Work out the finished part from the listing and answer in its coordinate system (mm). A direction names the side the tool comes from. Coordinates: 2 decimals unless noted, no trailing zeros. Write each loop counter-clockwise with the first axis right and the second up, starting at its lowest first coordinate (ties: lowest second). Pieces come first, ordered by that corner, then holes. Notation, with made-up numbers: (8, -37) - (30, -37) arc R13 cw to (30, -13) - close; hole circle Ø7 at (45, -7.75). An arc over 180 degrees is marked (long way). Use one line per item in the form item = value. Start each with the question number.
Item 1: A cutting plane is placed at B-B (z = 30). Write down the section's boundary in (x, y).
Item 2: Determine the mould class of faces 1 (the cylindrical face through (25.879, 48.412, 56.766)), 2 (the flat face through (36, 30.667, 5)), 3 (the cylindrical face through (26.91, 48.41, 2.12)) for opening direction X: released by +X, released by -X, zero draft, split by the parting line, or undercut.
Item 3: Given pin 1 (1.4 mm diameter, centred on y = 45, z = 51, fed in from +X); pin 2 (12 mm diameter, centred on y = 49, z = 39, fed in from +X); pin 3 (8 mm diameter, centred on x = 50, y = 36.5, fed in from -Z), each flat-ended and moving along its own axis, determine where each tip first touches the part or whether it passes through.
Item 4: For faces 4 (the flat face through (16.534, 48, 51)), 5 (the flat face through (36, 65.667, 5)), determine the directions among +Z, -Z, +X, -X, +Y, -Y from which every point of the face is accessible in a straight line to the end or side of a thin tool.
Item 5: Consider probe 1 along Z at (x, y) = (29.5, 34.5); probe 2 along Z at (x, y) = (23.5, 40); probe 3 along X at (y, z) = (38, 32). Determine where each line is inside the solid, lowest interval first.
Item 6: A cutting plane is placed at A-A (x = 40). Write down the section's boundary in (y, z).
from build123d import *

# Parameters (mm, degrees)
SKETCH_1_R      = 25.5
EXTRUDE_1_DEPTH = 35
CHAMFER_1_SIZE  = 1.5
FILLET_1_R      = 2
CHAMFER_2_SIZE  = 0.5


with BuildPart() as part:
    # Эскиз1 → Бобышка-Вытянуть1 (new body)
    # profile 1 of 3: a face of its own
    with BuildSketch(Plane(origin=(0, 65.667309681, 0), x_dir=(-1, 0, 0), z_dir=(0, -1, 0))):
        with BuildLine():
            ThreePointArc((-32.569554052, -57.83154498), (-26.905120992, -2.121558707), (-31.457793139, -57.933399285))
            Line((-31.457793139, -57.933399285), (-31.386430924, -56.935948818))
            ThreePointArc((-31.386430924, -56.935948818), (-26.058947255, -56.789767316), (-20.863962526, -55.599983748))
            Line((-20.863962526, -55.599983748), (-21.100431285, -54.895855797))
            ThreePointArc((-21.100431285, -54.895855797), (-26.672454195, -56.113662764), (-32.375987665, -56.099553559))
            Line((-32.375987665, -56.099553559), (-32.569554052, -57.83154498))
        make_face()
        with Locations((-29.45965114, -30.004786206)):
            Circle(SKETCH_1_R, mode=Mode.SUBTRACT)
    # profile 2 of 3: a face of its own
    with BuildSketch(Plane(origin=(0, 65.667309681, 0), x_dir=(-1, 0, 0), z_dir=(0, -1, 0))):
        with BuildLine():
            ThreePointArc((-42.146247167, -7.884653267), (-43.001975074, -8.397947879), (-43.836965332, -8.944329501))
            Line((-43.836965332, -8.944329501), (-42.312872357, -9.648278017))
            Line((-42.312872357, -9.648278017), (-42.146247167, -7.884653267))
        make_face()
    # profile 3 of 3: a face of its own
    with BuildSketch(Plane(origin=(0, 65.667309681, 0), x_dir=(-1, 0, 0), z_dir=(0, -1, 0))):
        with BuildLine():
            Line((-16.534234919, -50.219751552), (-16.534234919, -51.986224182))
            ThreePointArc((-16.534234919, -51.986224182), (-15.879111186, -51.587625096), (-15.236269322, -51.169507079))
            Line((-15.236269322, -51.169507079), (-16.534234919, -50.219751552))
        make_face()
    extrude(amount=EXTRUDE_1_DEPTH)

    # Фаска1
    # the kernel refuses this chamfer: 1.5 mm, written as the material it takes off along each edge
    with BuildSketch(Plane(origin=(32.569554052, 69.524834163, 57.83154498), x_dir=(0.9905736381961588, 0, -0.13698126627690838), z_dir=(0, -1, 0))) as chamfer_1_piece_1:
        with BuildLine():
            Line((1.462313623, 0), (CHAMFER_1_SIZE * 0.0261127432615, -CHAMFER_1_SIZE * 0.999659004181))
            Line((CHAMFER_1_SIZE * 0.0261127432615, -CHAMFER_1_SIZE * 0.999659004181), (0, 0))
            ThreePointArc((0, 0), (0.751799837, 0.009540273), (1.462313623, 0))
        make_face()
    extrude(amount=42.715048964, mode=Mode.SUBTRACT)

    # Скругление1
    fillet_1_edges = [part.edges().sort_by_distance(p)[0] for p in [
        (34.018083377, 48.167309681, 57.631235408),
    ]]
    fillet(fillet_1_edges, radius=FILLET_1_R)

    # Фаска2
    # the kernel refuses this chamfer: 0.5 mm, written as the material it takes off along each edge
    with BuildSketch(Plane(origin=(31.386430924, 66.965316212, 56.935948818), x_dir=(0.0713622142429535, 0, 0.9974504671302444), z_dir=(0, -1, 0))) as chamfer_2_piece_1:
        with BuildLine():
            Line((CHAMFER_2_SIZE, 0), (-0.004717821, 0.504717821))
            ThreePointArc((-0.004717821, 0.504717821), (-0.001247153, 0.259508631), (0, 0))
            Line((0, 0), (CHAMFER_2_SIZE, 0))
        make_face()
    extrude(amount=37.596013061, mode=Mode.SUBTRACT)


solid = part.part
Answer:
q1.outline = (1.46, 30.67) - (3.96, 30.67) - (3.96, 65.67) - (1.46, 65.67) - close; (54.96, 30.67) - (57.46, 30.67) - (57.46, 65.67) - (54.96, 65.67) - close
q2.face_1 = undercut
q2.face_2 = zero draft
q2.face_3 = split by the parting line
q3.pin_1 = 48.75
q3.pin_2 = 57.3
q3.pin_3 = 7.41
q4.face_4 = +Y, -Y
q4.face_5 = +Z, -Z, +X, -X, +Y
q5.probe_1 = 2 to 4.5, 55.5 to 56.26, 57 to 58
q5.probe_2 = 2.65 to 5.21, 54.8 to 55.58, 56.34 to 57.36
q5.probe_3 = 1.53 to 4.04, 54.88 to 57.39
q6.outline = (30.67, 4.06) - (65.67, 4.06) - (65.67, 6.79) - (30.67, 6.79) - close; (30.67, 53.22) - (65.67, 53.22) - (65.67, 55.95) - (30.67, 55.95) - close
